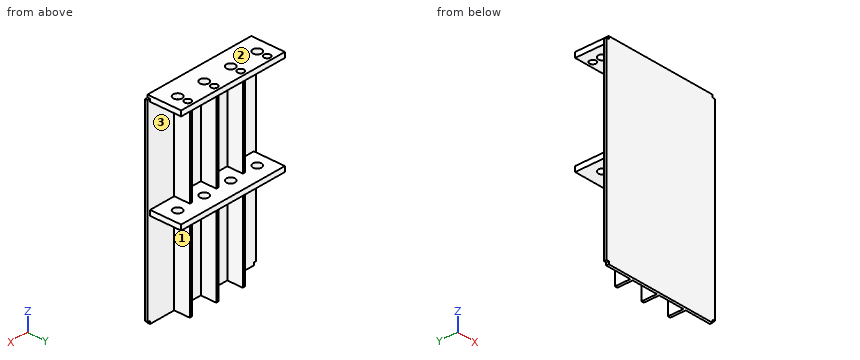
```python
from build123d import *

# Parameters (mm, degrees)
GEARBOX_MOUNT_DEPTH = 76
BOSS_EXTRUDE6_START = 37
SKETCH7_R           = 1.7
BOSS_EXTRUDE6_DEPTH = 1
BOSS_EXTRUDE7_START = 75
SKETCH8_R           = 1.7
SKETCH8_R_2         = 1.25
BOSS_EXTRUDE7_DEPTH = 1
SKETCH9_W           = 1
SKETCH9_H           = 1
CUT_EXTRUDE1_DEPTH  = 119.118983452


with BuildPart() as part:
    # Sketch2 → Gearbox Mount (new body)
    with BuildSketch(Plane.XY):
        Polygon((-24.506477671, 76.636122542), (-24.506477671, 70.636122542), (-14.306477671, 70.636122542), (-14.306477671, 76.636122542), (-13.306477671, 76.636122542), (-13.306477671, 70.636122542), (-3.106477671, 70.636122542), (-3.106477671, 76.636122542), (-2.106477671, 76.636122542), (-2.106477671, 70.636122542), (8.093522329, 70.636122542), (9.093522329, 70.636122542), (9.093522329, 69.636122542), (-36.706477671, 69.636122542), (-36.706477671, 70.636122542), (-35.706477671, 70.636122542), (-25.506477671, 70.636122542), (-25.506477671, 76.636122542), align=None)
    extrude(amount=GEARBOX_MOUNT_DEPTH)

    # Sketch7 → Boss-Extrude6 (add, symmetric)
    with BuildSketch(Plane.XY.offset(BOSS_EXTRUDE6_START)):
        Polygon((-24.506477671, 76.636122542), (-24.506477671, 70.636122542), (-14.306477671, 70.636122542), (-14.306477671, 76.636122542), (-13.306477671, 76.636122542), (-13.306477671, 70.636122542), (-3.106477671, 70.636122542), (-3.106477671, 76.636122542), (-2.106477671, 76.636122542), (-2.106477671, 70.636122542), (8.093522329, 70.636122542), (8.093522329, 82.636122542), (-35.706477671, 82.636122542), (-35.706477671, 70.636122542), (-25.506477671, 70.636122542), (-25.506477671, 76.636122542), align=None)
        with Locations((-19.406477671, 76.636122542)):
            Circle(SKETCH7_R, mode=Mode.SUBTRACT)
        with Locations((-30.606477671, 76.636122542)):
            Circle(SKETCH7_R, mode=Mode.SUBTRACT)
        with Locations((-8.206477671, 76.636122542)):
            Circle(SKETCH7_R, mode=Mode.SUBTRACT)
        with Locations((2.993522329, 76.636122542)):
            Circle(SKETCH7_R, mode=Mode.SUBTRACT)
    extrude(amount=BOSS_EXTRUDE6_DEPTH, both=True)

    # Sketch8 → Boss-Extrude7 (add, symmetric)
    with BuildSketch(Plane.XY.offset(BOSS_EXTRUDE7_START)):
        Polygon((-35.706477671, 82.636122542), (-35.706477671, 70.636122542), (-25.506477671, 70.636122542), (-25.506477671, 76.636122542), (-24.506477671, 76.636122542), (-24.506477671, 70.636122542), (-14.306477671, 70.636122542), (-14.306477671, 76.636122542), (-13.306477671, 76.636122542), (-13.306477671, 70.636122542), (-3.106477671, 70.636122542), (-3.106477671, 76.636122542), (-2.106477671, 76.636122542), (-2.106477671, 70.636122542), (8.093522329, 70.636122542), (8.093522329, 82.636122542), align=None)
        with Locations((-30.606477671, 76.636122542)):
            Circle(SKETCH8_R, mode=Mode.SUBTRACT)
        with Locations((-30.606477671, 80.486122542)):
            Circle(SKETCH8_R_2, mode=Mode.SUBTRACT)
        with Locations((-19.406477671, 80.486122542)):
            Circle(SKETCH8_R_2, mode=Mode.SUBTRACT)
        with Locations((-19.406477671, 76.636122542)):
            Circle(SKETCH8_R, mode=Mode.SUBTRACT)
        with Locations((-8.206477671, 80.486122542)):
            Circle(SKETCH8_R_2, mode=Mode.SUBTRACT)
        with Locations((-8.206477671, 76.636122542)):
            Circle(SKETCH8_R, mode=Mode.SUBTRACT)
        with Locations((2.993522329, 80.486122542)):
            Circle(SKETCH8_R_2, mode=Mode.SUBTRACT)
        with Locations((2.993522329, 76.636122542)):
            Circle(SKETCH8_R, mode=Mode.SUBTRACT)
    extrude(amount=BOSS_EXTRUDE7_DEPTH, both=True)

    # Sketch9 → Cut-Extrude1 (cut, through all)
    with BuildSketch(Plane(origin=(0, 0, 0), x_dir=(1, 0, 0), z_dir=(0, 1, 0))):
        with Locations((-36.206477671, -0.5)):
            Rectangle(SKETCH9_W, SKETCH9_H)
        with Locations((8.593522329, -0.5)):
            Rectangle(SKETCH9_W, SKETCH9_H)
        with Locations((8.593522329, -75.5)):
            Rectangle(SKETCH9_W, SKETCH9_H)
        with Locations((-36.206477671, -75.5)):
            Rectangle(SKETCH9_W, SKETCH9_H)
    extrude(amount=CUT_EXTRUDE1_DEPTH, mode=Mode.SUBTRACT)


solid = part.part
```
Geometry: final body of the model. Coordinates: model frame, mm. Face numbers are marked on the shaded views. A direction names the side the tool comes from. Round coordinates to 2 decimals unless told otherwise and drop trailing zeros. Write each loop counter-clockwise with the first axis right and the second up, starting at its lowest first coordinate (ties: lowest second). Pieces come first, ordered by that corner, then holes. Notation, with made-up numbers: (20.25, 7) -> (74.25, 7) arc R28 ccw to (74.25, 30) -> close; hole circle Ø3 at (43.5, -34). An arc over 180 degrees is marked (long way). Use CSV: the item, a comma, the result in double quotes. Start each with the question number.
Q1. Line query: L1, parallel to X at y = 76.5, z = 18.5; L2, parallel to Z at x = -13, y = 79.25; L3, parallel to Y at x = -12.5, z = 32.5. Output: solid intervals per line, ascending.
Q2. Section B-B (y = 71.75). Give the number of separate pieces and of enclosed holes in the cut face, plus the area to 3 significant figures.
Q3. Reachability of the marked faces 1, 2 and 3 from +Z, -Z, +X, -X, +Y, -Y: full face, straight path, thin tool, end or side. Return the list, or none.
Q4. Section A-A (z = 50). Return loops of the section in (x, y).
Q5. First-contact query: pin 1 Ø3 at (x, z) = (-9.5, 25.5) entering from +Y; pin 2 Ø0.5 at (x, z) = (-2.5, 16) entering from +Y; pin 3 Ø4 at (x, y) = (-8.21, 76.64) entering from -Z; pin 4 Ø6 at (y, z) = (80.5, 15) entering from -X. Flat tips, straight axial feed; report the tip coordinate or a pass-through.
Q6. Section C-C (x = -5). Return loops of the section in (y, z), plus the area to 3 significant figures.
Result sheet:
1,L1,"-25.51 to -24.51, -14.31 to -13.31, -3.11 to -2.11"
1,L2,"36 to 38, 74 to 76"
1,L3,"69.64 to 70.64"
2,separate pieces,"1"
2,enclosed holes,"2"
2,area,"391 mm²"
3,face 1,"-Z, +X, +Y"
3,face 2,"+Z, +X, -X, +Y, -Y"
3,face 3,"+X, +Y"
4,outline,"(-36.71, 69.64) -> (9.09, 69.64) -> (9.09, 70.64) -> (-2.11, 70.64) -> (-2.11, 76.64) -> (-3.11, 76.64) -> (-3.11, 70.64) -> (-13.31, 70.64) -> (-13.31, 76.64) -> (-14.31, 76.64) -> (-14.31, 70.64) -> (-24.51, 70.64) -> (-24.51, 76.64) -> (-25.51, 76.64) -> (-25.51, 70.64) -> (-36.71, 70.64) -> close"
5,pin 1,"y = 70.64"
5,pin 2,"y = 76.64"
5,pin 3,"z = 36"
5,pin 4,"through"
6,outline,"(69.64, 0) -> (70.64, 0) -> (70.64, 36) -> (82.64, 36) -> (82.64, 38) -> (70.64, 38) -> (70.64, 74) -> (82.64, 74) -> (82.64, 76) -> (69.64, 76) -> close"
6,area,"124 mm²"
